Can you work these out from the drawing? Everything is in mm from the part's minimum corner. Coordinates: 2 decimals unless noted, no trailing zeros. Order: outer loops, then holes, each group sorted by start corner. A loop starts at its lowest first (then second) coordinate and runs counter-clockwise, first axis right, second up. Notation, with made-up numbers: (-12, 63) - (7, 63) arc R22 ccw to (7, 92) - close; hole circle Ø7 at (-36, 12.5). An arc over 180 degrees is marked (long way). Use a Markdown table: item, result. Add a question column.
(1) I want a section at B-B (z = 20.5). List the corners of the cut face in (x, y) for me, and give its area (3 significant figures).
(2) For pin 1 Ø2 at (x, y) = (239, 7) entering from -Z; pin 2 Ø3 at (x, y) = (16, 6.5) entering from +Z; pin 3 Ø3 at (y, z) = (6.5, 123.5) entering from +X, each with a flat end and sliding along its axis, tell me the tip position at first contact or that it passes through.
(3) I want a section at C-C (x = 55). List the corners of the cut face in (y, z) for me.
(4) We'd pull the mould along Y, two halves only. Please class the marked faces 1 and 2: pulls with the +Y half, pulls with the -Y half, needs draft (parallel to the pull), parting line crosses it, or undercut.
(5) If I drill on L1, parallel to Z at x = 354, y = 3.5; L2, parallel to X at y = 8.25, z = 123; L3, parallel to X at y = 5.25, z = 41, over which ranges is the centre line in solid material (lowest first)? Write a range as [from, to].
(6) I want a section at A-A (y = 4.25). List the corners of the cut face in (x, z) for me, and give its area (4 significant figures).
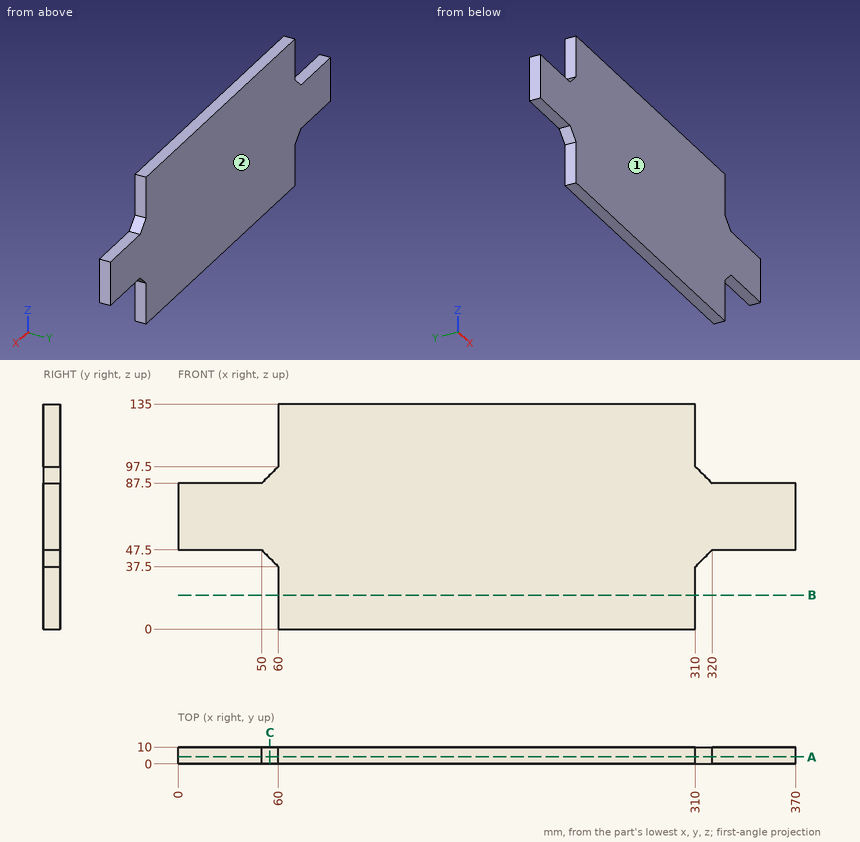
Answers follow:
| question | item | result |
|---|---|---|
| 1 | outline | (60, 0) - (310, 0) - (310, 10) - (60, 10) - close |
| 1 | area | 2,500 mm² |
| 2 | pin 1 | stops at z = 0 |
| 2 | pin 2 | stops at z = 87.5 |
| 2 | pin 3 | stops at x = 310 |
| 3 | outline | (0, 42.5) - (10, 42.5) - (10, 92.5) - (0, 92.5) - close |
| 4 | face 1 | pulls with the -Y half |
| 4 | face 2 | pulls with the +Y half |
| 5 | L1 | z = [47.5, 87.5] |
| 5 | L2 | x = [60, 310] |
| 5 | L3 | x = [56.5, 313.5] |
| 6 | outline | (0, 47.5) - (50, 47.5) - (60, 37.5) - (60, 0) - (310, 0) - (310, 37.5) - (320, 47.5) - (370, 47.5) - (370, 87.5) - (320, 87.5) - (310, 97.5) - (310, 135) - (60, 135) - (60, 97.5) - (50, 87.5) - (0, 87.5) - close |
| 6 | area | 38,750 mm² |
